Check sheet for the modelled part. Datum: model origin and axes. Units: mm. Face numbers are marked on the shaded views. A direction names the side the tool comes from. Round coordinates to 2 decimals unless told otherwise and drop trailing zeros. Loops run counter-clockwise (first coordinate to the right, second up) from the corner with the lowest first, then second, coordinate; pieces in that order, holes last. Notation, with made-up numbers: M -7,49.5 L 24,49.5 A8 ccw 24,64.5 Z; hole C -16.5,77 d2. An arc over 180 degrees is marked long. One line per question, with ' | ' between items. Start each with the question number.
(1) Section check B-B (y = 17.25). Record the boundary of the cut face in (x, z), and give its area (3 significant figures).
(2) Thickness scan on probe 1 along Z at (x, y) = (12.5, 12.7); probe 2 along X at (y, z) = (18.25, 10.5); probe 3 along X at (y, z) = (24.25, 22). Record the ranges inside material, lowest first. Write a range as [from, to].
(3) Section check C-C (x = -24). Record the boundary of the cut face in (y, z), and give its area (3 significant figures).
(4) Tool access check on the marked faces 1, 2 and 3. Record the directions out of +Z, -Z, +X, -X, +Y, -Y that give a thin tool (end or side, any length) a straight path to the whole face; none if there is none.
(5) Go/stop test with flat-tipped pins: P1, Ø10, axis at x = -19.07, y = 12.7, coming from the -Z side; P2, Ø5, axis at x = 16.5, y = 9.5, coming from the +Z side; P3, Ø12, axis at y = 10.5, z = 37.5, coming from the +X side; P4, Ø12, axis at y = 19.5, z = 23.5, coming from the -X side. Record where each tip stops, or that it passes through.
(6) Section check A-A (z = 5). Record the boundary of the cut face in (x, y), and give its area (3 significant figures).
(7) Draft check along X on the marked faces 4, 5 and 6. Enter one of: +X half, -X half, draft (parallel to the pull), parting line (faces both ways), or undercut.
(8) Section check D-D (z = 31). Record the boundary of the cut face in (x, y).
```python
from build123d import *

# Parameters (mm, degrees)
F0_W     = 76.2
F0_H     = 25.4
F0_R     = 6.35
F1_DEPTH = 12.7
F3_DEPTH = 12.7
F4_W     = 25.4
F4_H     = 25.4
F5_DEPTH = 44.45
F7_DEPTH = 25.4
F8_R     = 6.35
F9_DEPTH = 25.4


with BuildPart() as f1:
    # F0 (on Top) → F1 (new body)
    with BuildSketch(Plane.XY):
        with Locations((6.3257696523, 12.7)):
            Rectangle(F0_W, F0_H)
        with Locations((-19.0742303477, 12.7)):
            Circle(F0_R, mode=Mode.SUBTRACT)
        with Locations((31.7257696523, 12.7)):
            Circle(F0_R, mode=Mode.SUBTRACT)
    extrude(amount=F1_DEPTH)

    # F2 (on face) → F3 (cut)
    with BuildSketch(Plane.XY.offset(12.7)):
        with BuildLine():
            ThreePointArc((-19.4995366037, 0), (-31.2612298583, 12.4208945177), (-20.1185699552, 25.4))
            Line((-20.1185699552, 25.4), (-31.7742303477, 25.4))
            Line((-31.7742303477, 25.4), (-31.7742303477, 0))
            Line((-31.7742303477, 0), (-19.4995366037, 0))
        make_face()
        with BuildLine():
            Line((44.4257696523, 25.4), (32.7468659845, 25.4))
            ThreePointArc((32.7468659845, 25.4), (40.454102952, 22.0844190513), (44.4257696523, 14.6938546396))
            Line((44.4257696523, 14.6938546396), (44.4257696523, 25.4))
        make_face()
        with BuildLine():
            ThreePointArc((44.4257696523, 10.701621252), (40.4769444267, 3.3320470648), (32.8087434173, 0))
            Line((32.8087434173, 0), (44.4257696523, 0))
            Line((44.4257696523, 0), (44.4257696523, 10.701621252))
        make_face()
    extrude(amount=-F3_DEPTH, mode=Mode.SUBTRACT)

    # F4 (on Top) → F5 (join)
    with BuildSketch(Plane.XY):
        with Locations((6.41142525, 12.7)):
            Rectangle(F4_W, F4_H)
    extrude(amount=F5_DEPTH)

    # F6 (on face) → F7 (cut)
    with BuildSketch(Plane(origin=(-6.28857475, 0, 0), x_dir=(0, -1, 0), z_dir=(-1, 0, 0))):
        with BuildLine():
            ThreePointArc((-25.4, 31.75), (-21.6802561211, 40.7302561211), (-12.7, 44.45))
            Line((-12.7, 44.45), (-25.4, 44.45))
            Line((-25.4, 44.45), (-25.4, 31.75))
        make_face()
        with BuildLine():
            ThreePointArc((-12.7, 44.45), (-3.7197438789, 40.7302561211), (0, 31.75))
            Line((0, 31.75), (0, 44.45))
            Line((0, 44.45), (-12.7, 44.45))
        make_face()
    extrude(amount=-F7_DEPTH, mode=Mode.SUBTRACT)

    # F8 (on face) → F9 (cut)
    with BuildSketch(Plane(origin=(-6.28857475, 0, 0), x_dir=(0, -1, 0), z_dir=(-1, 0, 0))):
        with Locations((-12.7, 31.75)):
            Circle(F8_R)
    extrude(amount=-F9_DEPTH, mode=Mode.SUBTRACT)


solid = f1.part
```
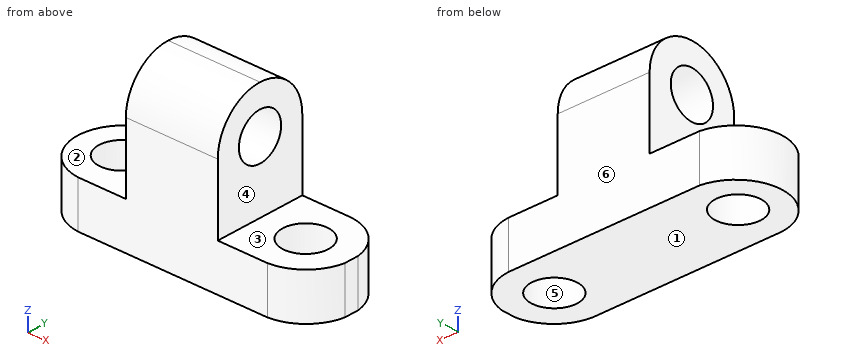
The answers:
1) outline: M -30.44,0 L -23.5,0 L -23.5,12.7 L -30.44,12.7 Z; M -14.64,0 L 27.3,0 L 27.3,12.7 L 19.11,12.7 L 19.11,27.32 L -6.29,27.32 L -6.29,12.7 L -14.64,12.7 Z; M -6.29,36.18 L 19.11,36.18 L 19.11,43.61 L -6.29,43.61 Z; M 36.16,0 L 43.74,0 L 43.74,12.7 L 36.16,12.7 Z | area: 1,280 mm²
2) probe 1: [0, 25.4], [38.1, 44.45] | probe 2: [-30.01, -22.16], [-15.99, 28.64], [34.81, 43.31] | probe 3: [-6.29, 19.11]
3) outline: M 1.21,0 L 8.69,0 L 8.69,12.7 L 1.21,12.7 Z; M 16.71,0 L 24.26,0 L 24.26,12.7 L 16.71,12.7 Z | area: 191 mm²
4) face 1: -Z, +X, -X, +Y, -Y | face 2: +Z, -X, +Y, -Y | face 3: +Z, +X, +Y, -Y
5) P1: through | P2: z = 44.43 | P3: x = 19.11 | P4: x = -6.29
6) outline: M -20.12,25.4 A12.77 ccw -19.5,0 L 32.81,0 A12.73 ccw 44.43,10.7 L 44.43,14.69 A12.73 ccw 32.75,25.4 Z; hole C -19.07,12.7 d12.7; hole C 31.73,12.7 d12.7 | area: 1,540 mm²
7) face 4: +X half | face 5: undercut | face 6: draft
8) outline: M -6.29,0 L 19.11,0 L 19.11,6.39 L -6.29,6.39 Z; M -6.29,19.01 L 19.11,19.01 L 19.11,25.4 L -6.29,25.4 Z
